Input: part model. Units: mm. Frame: model coordinates. A direction names the side the tool comes from. Give positions to 0.01 mm unless a question says otherwise; leave off trailing zeros. Loops run counter-clockwise (first coordinate to the right, second up) from the corner with the lowest first, then second, coordinate; pieces in that order, holes last. Notation, with made-up numbers: M 15,43.25 L 38,43.25 A17 ccw 38,58.25 Z; hole C 14.5,-27 d5. An arc over 180 degrees is marked long. Answer as a JSON object with one key per item and string values. Group by question number.
```python
from build123d import *

# Parameters (mm, degrees)
F1_DEPTH = 25
F2_W     = 2.9
F2_H     = 10
F3_DEPTH = 10
F4_R     = 1.5
F5_DEPTH = 9
F6_SIZE  = 2


with BuildPart() as f1:
    # F0 (on Right) → F1 (new body)
    with BuildSketch(Plane.YZ):
        Polygon((-24, 0), (0, 0), (0, 4), (-20, 4), (-20, 12), (0, 12), (0, 16), (-24, 16), align=None)
    extrude(amount=F1_DEPTH)

    # F2 (on face) → F3 (join)
    with BuildSketch(Plane.XZ.offset(24)):
        with Locations((9.5, 8)):
            Rectangle(F2_W, F2_H)
        with Locations((15.5, 8)):
            Rectangle(F2_W, F2_H)
    extrude(amount=F3_DEPTH)

    # F4 (on face) → F5 (cut)
    with BuildSketch(Plane.YZ.offset(16.95)):
        with BuildLine():
            ThreePointArc((-34, 8), (-32.535534, 11.535534), (-29, 13))
            Line((-29, 13), (-34, 13))
            Line((-34, 13), (-34, 8))
        make_face()
        with BuildLine():
            ThreePointArc((-29, 3), (-32.535534, 4.464466), (-34, 8))
            Line((-34, 8), (-34, 3))
            Line((-34, 3), (-29, 3))
        make_face()
        with Locations((-29, 8)):
            Circle(F4_R)
    extrude(amount=-F5_DEPTH, mode=Mode.SUBTRACT)

    # F6
    f6_edges = [f1.edges().sort_by_distance(p)[0] for p in [
        (12.5, 0, 12),
        (12.5, 0, 4),
    ]]
    chamfer(f6_edges, length=F6_SIZE)


solid = f1.part
```
1. Material intervals for L1, parallel to Z at x = 10.2, y = -29; L2, parallel to Z at x = 16.5, y = -16.5; L3, parallel to Y at x = 21.5, z = 14.25, sorted ascending.
2. Section B-B (x = 9.75). Output: boundary loops of the cut face in (y, z), then the cut area to 3 significant figures.
3. Section A-A (y = -14). Output: boundary loops of the cut face in (x, z), then the cut area to 3 significant figures.
4. Section D-D (y = -28.5). Output: boundary loops of the cut face in (x, z).
5. First-contact query: P1, Ø5, axis at y = -28, z = 8, coming from the +X side; P2, Ø1.4, axis at x = 9.5, y = -26.5, coming from the +Z side; P3, Ø5, axis at x = 6, z = 6, coming from the +Y side; P4, Ø8, axis at y = -16.5, z = 13, coming from the -X side. Flat tips, straight axial feed; report the tip coordinate or a pass-through.
6. Reachability of faces 1 (the flat face through (16.95, -27.8, 6.8)), 2 (the flat face through (10.95, -27.8, 6.8)), 3 (the flat face through (8.05, -27.8, 6.8)), 4 (the flat face through (12, -1, 13)), 5 (the flat face through (15, -26, 3)) from +Z, -Z, +X, -X, +Y, -Y: full face, straight path, thin tool, end or side. Return the list, or none.
7. Mould query, pull axis Y, two halves, no side actions, for faces 6 (the flat face through (0, -15, 3)), 7 (the flat face through (12, 0, 1)), 8 (the cylindrical face through (15.52, -30.5, 8.07)). Classes: pulls with the +Y half, pulls with the -Y half, needs draft (parallel to the pull), parting line crosses it, or undercut.
8. Section C-C (x = 1.75). Output: boundary loops of the cut face in (y, z).
Geometry results:
{
 "1": {"L1": "3 to 6.5, 9.5 to 13", "L2": "0 to 4, 12 to 16", "L3": "-24 to 0"},
 "2": {"outline": "M -29,3 L -24,3 L -24,0 L 0,0 L 0,2 L -2,4 L -20,4 L -20,12 L -2,12 L 0,14 L 0,16 L -24,16 L -24,13 L -29,13 A5 ccw Z; hole C -29,8 d3", "area": "302 mm2"},
 "3": {"outline": "M 0,0 L 25,0 L 25,4 L 0,4 Z; M 0,12 L 25,12 L 25,16 L 0,16 Z", "area": "200 mm2"},
 "4": {"outline": "M 8.05,3 L 10.95,3 L 10.95,6.59 L 8.05,6.59 Z; M 8.05,9.41 L 10.95,9.41 L 10.95,13 L 8.05,13 Z; M 14.05,3 L 16.95,3 L 16.95,6.59 L 14.05,6.59 Z; M 14.05,9.41 L 16.95,9.41 L 16.95,13 L 14.05,13 Z"},
 "5": {"P1": "x = 16.95", "P2": "z = 13", "P3": "y = -1.5", "P4": "x = 0"},
 "6": {"face 1": "+Z, -Z, +X, -Y", "face 2": "+Z, -Z, -Y", "face 3": "+Z, -Z, -X, -Y", "face 4": "+X, -X, +Y", "face 5": "-Z, +X, -X, -Y"},
 "7": {"face 6": "needs draft", "face 7": "pulls with the +Y half", "face 8": "undercut"},
 "8": {"outline": "M -24,0 L 0,0 L 0,2 L -2,4 L -20,4 L -20,12 L -2,12 L 0,14 L 0,16 L -24,16 Z"}
}
